```python
from build123d import *

# Parameters (mm, degrees)
SKETCH1_W                             = 12.7
SKETCH1_H                             = 50.8
BOSS_EXTRUDE1_DEPTH                   = 228.6
F_1_4_20_TAPPED_HOLE1_D               = 5.1054
F_1_4_20_TAPPED_HOLE1_DEPTH           = 19.05
F_1_4_20_TAPPED_HOLE1_TIP             = 1.533816902
F_1_4_20_TAPPED_HOLE1_ON_FACE_2_D     = 5.1054
F_1_4_20_TAPPED_HOLE1_ON_FACE_2_DEPTH = 19.05
F_1_4_20_TAPPED_HOLE1_ON_FACE_2_TIP   = 1.533816902
CUT_EXTRUDE1_DEPTH                    = 9.525
CUT_EXTRUDE2_DEPTH                    = 235.370061281
CUT_EXTRUDE3_DEPTH                    = 235.52055347


with BuildPart() as part:
    # Sketch1 → Boss-Extrude1 (new, symmetric)
    with BuildSketch(Plane(origin=(0, 0, 0), x_dir=(0, 0, -1), z_dir=(1, 0, 0))):
        with Locations((6.35, 25.4)):
            Rectangle(SKETCH1_W, SKETCH1_H)
    extrude(amount=BOSS_EXTRUDE1_DEPTH, both=True)

    # 1/4-20 Tapped Hole1
    with Locations(Plane(origin=(228.6, 41.275, -6.35), x_dir=(0, 0, 1), z_dir=(1, 0, 0))):
        with Locations((0, 0), (0, 31.75)):
            Hole(F_1_4_20_TAPPED_HOLE1_D / 2, depth=F_1_4_20_TAPPED_HOLE1_DEPTH)
            with Locations((0, 0, -(F_1_4_20_TAPPED_HOLE1_DEPTH + F_1_4_20_TAPPED_HOLE1_TIP / 2))):  # 118° drill point
                Cone(0, F_1_4_20_TAPPED_HOLE1_D / 2, F_1_4_20_TAPPED_HOLE1_TIP, mode=Mode.SUBTRACT)

    # 1/4-20 Tapped Hole1 on face 2
    with Locations(Plane(origin=(-228.6, 9.525, -6.35), x_dir=(0, 0, -1), z_dir=(-1, 0, 0))):
        with Locations((0, 0), (0, -31.75)):
            Hole(F_1_4_20_TAPPED_HOLE1_ON_FACE_2_D / 2, depth=F_1_4_20_TAPPED_HOLE1_ON_FACE_2_DEPTH)
            with Locations((0, 0, -(F_1_4_20_TAPPED_HOLE1_ON_FACE_2_DEPTH + F_1_4_20_TAPPED_HOLE1_ON_FACE_2_TIP / 2))):  # 118° drill point
                Cone(0, F_1_4_20_TAPPED_HOLE1_ON_FACE_2_D / 2, F_1_4_20_TAPPED_HOLE1_ON_FACE_2_TIP, mode=Mode.SUBTRACT)

    # Sketch4 → Cut-Extrude1 (cut)
    with BuildSketch(Plane(origin=(0, 0, -12.7), x_dir=(-1, 0, 0), z_dir=(0, 0, -1))):
        with BuildLine():
            Line((200.025, 47.625), (-200.025, 47.625))
            ThreePointArc((-200.025, 47.625), (-202.27006403, 46.69506403), (-203.2, 44.45))
            Line((-203.2, 44.45), (-203.2, 6.35))
            ThreePointArc((-203.2, 6.35), (-202.27006403, 4.10493597), (-200.025, 3.175))
            Line((-200.025, 3.175), (200.025, 3.175))
            ThreePointArc((200.025, 3.175), (202.27006403, 4.10493597), (203.2, 6.35))
            Line((203.2, 6.35), (203.2, 44.45))
            ThreePointArc((203.2, 44.45), (202.27006403, 46.69506403), (200.025, 47.625))
        make_face()
    extrude(amount=-CUT_EXTRUDE1_DEPTH, mode=Mode.SUBTRACT)

    # Sketch5 → Cut-Extrude2 (cut, through all)
    with BuildSketch(Plane(origin=(0, 0, -3.175), x_dir=(-1, 0, 0), z_dir=(0, 0, -1))):
        with BuildLine():
            Line((-200.025, 41.275), (-200.025, 9.525))
            ThreePointArc((-200.025, 9.525), (-199.09506403, 7.27993597), (-196.85, 6.35))
            Line((-196.85, 6.35), (-172.079670497, 6.35))
            ThreePointArc((-172.079670497, 6.35), (-169.226482862, 8.132180803), (-169.576379466, 11.477987203))
            Line((-169.576379466, 11.477987203), (-194.346708969, 43.227987203))
            ThreePointArc((-194.346708969, 43.227987203), (-197.882636426, 44.277380224), (-200.025, 41.275))
        make_face()
        with BuildLine():
            Line((-183.245495534, 39.322012797), (-158.475166031, 7.572012797))
            ThreePointArc((-158.475166031, 7.572012797), (-154.939238574, 6.522619776), (-152.796875, 9.525))
            Line((-152.796875, 9.525), (-152.796875, 41.275))
            ThreePointArc((-152.796875, 41.275), (-153.72681097, 43.52006403), (-155.971875, 44.45))
            Line((-155.971875, 44.45), (-180.742204503, 44.45))
            ThreePointArc((-180.742204503, 44.45), (-183.595392138, 42.667819197), (-183.245495534, 39.322012797))
        make_face()
        with BuildLine():
            Line((-149.621875, 41.275), (-149.621875, 9.525))
            ThreePointArc((-149.621875, 9.525), (-148.69193903, 7.27993597), (-146.446875, 6.35))
            Line((-146.446875, 6.35), (-121.676545497, 6.35))
            ThreePointArc((-121.676545497, 6.35), (-118.823357862, 8.132180803), (-119.173254466, 11.477987203))
            Line((-119.173254466, 11.477987203), (-143.943583969, 43.227987203))
            ThreePointArc((-143.943583969, 43.227987203), (-147.479511426, 44.277380224), (-149.621875, 41.275))
        make_face()
        with BuildLine():
            Line((-132.842370534, 39.322012797), (-108.072041031, 7.572012797))
            ThreePointArc((-108.072041031, 7.572012797), (-104.536113574, 6.522619776), (-102.39375, 9.525))
            Line((-102.39375, 9.525), (-102.39375, 41.275))
            ThreePointArc((-102.39375, 41.275), (-103.32368597, 43.52006403), (-105.56875, 44.45))
            Line((-105.56875, 44.45), (-130.339079503, 44.45))
            ThreePointArc((-130.339079503, 44.45), (-133.192267138, 42.667819197), (-132.842370534, 39.322012797))
        make_face()
        with BuildLine():
            Line((-99.21875, 41.275), (-99.21875, 9.525))
            ThreePointArc((-99.21875, 9.525), (-98.28881403, 7.27993597), (-96.04375, 6.35))
            Line((-96.04375, 6.35), (-71.273420497, 6.35))
            ThreePointArc((-71.273420497, 6.35), (-68.420232862, 8.132180803), (-68.770129466, 11.477987203))
            Line((-68.770129466, 11.477987203), (-93.540458969, 43.227987203))
            ThreePointArc((-93.540458969, 43.227987203), (-97.076386426, 44.277380224), (-99.21875, 41.275))
        make_face()
        with BuildLine():
            Line((-82.439245534, 39.322012797), (-57.668916031, 7.572012797))
            ThreePointArc((-57.668916031, 7.572012797), (-54.132988574, 6.522619776), (-51.990625, 9.525))
            Line((-51.990625, 9.525), (-51.990625, 41.275))
            ThreePointArc((-51.990625, 41.275), (-52.92056097, 43.52006403), (-55.165625, 44.45))
            Line((-55.165625, 44.45), (-79.935954503, 44.45))
            ThreePointArc((-79.935954503, 44.45), (-82.789142138, 42.667819197), (-82.439245534, 39.322012797))
        make_face()
        with BuildLine():
            Line((-48.815625, 41.275), (-48.815625, 9.525))
            ThreePointArc((-48.815625, 9.525), (-47.88568903, 7.27993597), (-45.640625, 6.35))
            Line((-45.640625, 6.35), (-20.870295497, 6.35))
            ThreePointArc((-20.870295497, 6.35), (-18.017107862, 8.132180803), (-18.367004466, 11.477987203))
            Line((-18.367004466, 11.477987203), (-43.137333969, 43.227987203))
            ThreePointArc((-43.137333969, 43.227987203), (-46.673261426, 44.277380224), (-48.815625, 41.275))
        make_face()
        with BuildLine():
            Line((-32.036120534, 39.322012797), (-7.265791031, 7.572012797))
            ThreePointArc((-7.265791031, 7.572012797), (-3.729863574, 6.522619776), (-1.5875, 9.525))
            Line((-1.5875, 9.525), (-1.5875, 41.275))
            ThreePointArc((-1.5875, 41.275), (-2.51743597, 43.52006403), (-4.7625, 44.45))
            Line((-4.7625, 44.45), (-29.532829503, 44.45))
            ThreePointArc((-29.532829503, 44.45), (-32.386017138, 42.667819197), (-32.036120534, 39.322012797))
        make_face()
        with BuildLine():
            Line((1.5875, 41.275), (1.5875, 9.525))
            ThreePointArc((1.5875, 9.525), (2.51743597, 7.27993597), (4.7625, 6.35))
            Line((4.7625, 6.35), (29.532829503, 6.35))
            ThreePointArc((29.532829503, 6.35), (32.386017138, 8.132180803), (32.036120534, 11.477987203))
            Line((32.036120534, 11.477987203), (7.265791031, 43.227987203))
            ThreePointArc((7.265791031, 43.227987203), (3.729863574, 44.277380224), (1.5875, 41.275))
        make_face()
        with BuildLine():
            Line((18.367004466, 39.322012797), (43.137333969, 7.572012797))
            ThreePointArc((43.137333969, 7.572012797), (46.673261426, 6.522619776), (48.815625, 9.525))
            Line((48.815625, 9.525), (48.815625, 41.275))
            ThreePointArc((48.815625, 41.275), (47.88568903, 43.52006403), (45.640625, 44.45))
            Line((45.640625, 44.45), (20.870295497, 44.45))
            ThreePointArc((20.870295497, 44.45), (18.017107862, 42.667819197), (18.367004466, 39.322012797))
        make_face()
        with BuildLine():
            Line((51.990625, 41.275), (51.990625, 9.525))
            ThreePointArc((51.990625, 9.525), (52.92056097, 7.27993597), (55.165625, 6.35))
            Line((55.165625, 6.35), (79.935954503, 6.35))
            ThreePointArc((79.935954503, 6.35), (82.789142138, 8.132180803), (82.439245534, 11.477987203))
            Line((82.439245534, 11.477987203), (57.668916031, 43.227987203))
            ThreePointArc((57.668916031, 43.227987203), (54.132988574, 44.277380224), (51.990625, 41.275))
        make_face()
        with BuildLine():
            Line((68.770129466, 39.322012797), (93.540458969, 7.572012797))
            ThreePointArc((93.540458969, 7.572012797), (97.076386426, 6.522619776), (99.21875, 9.525))
            Line((99.21875, 9.525), (99.21875, 41.275))
            ThreePointArc((99.21875, 41.275), (98.28881403, 43.52006403), (96.04375, 44.45))
            Line((96.04375, 44.45), (71.273420497, 44.45))
            ThreePointArc((71.273420497, 44.45), (68.420232862, 42.667819197), (68.770129466, 39.322012797))
        make_face()
        with BuildLine():
            Line((102.39375, 41.275), (102.39375, 9.525))
            ThreePointArc((102.39375, 9.525), (103.32368597, 7.27993597), (105.56875, 6.35))
            Line((105.56875, 6.35), (130.339079503, 6.35))
            ThreePointArc((130.339079503, 6.35), (133.192267138, 8.132180803), (132.842370534, 11.477987203))
            Line((132.842370534, 11.477987203), (108.072041031, 43.227987203))
            ThreePointArc((108.072041031, 43.227987203), (104.536113574, 44.277380224), (102.39375, 41.275))
        make_face()
        with BuildLine():
            Line((119.173254466, 39.322012797), (143.943583969, 7.572012797))
            ThreePointArc((143.943583969, 7.572012797), (147.479511426, 6.522619776), (149.621875, 9.525))
            Line((149.621875, 9.525), (149.621875, 41.275))
            ThreePointArc((149.621875, 41.275), (148.69193903, 43.52006403), (146.446875, 44.45))
            Line((146.446875, 44.45), (121.676545497, 44.45))
            ThreePointArc((121.676545497, 44.45), (118.823357862, 42.667819197), (119.173254466, 39.322012797))
        make_face()
        with BuildLine():
            Line((152.796875, 41.275), (152.796875, 9.525))
            ThreePointArc((152.796875, 9.525), (153.72681097, 7.27993597), (155.971875, 6.35))
            Line((155.971875, 6.35), (180.742204503, 6.35))
            ThreePointArc((180.742204503, 6.35), (183.595392138, 8.132180803), (183.245495534, 11.477987203))
            Line((183.245495534, 11.477987203), (158.475166031, 43.227987203))
            ThreePointArc((158.475166031, 43.227987203), (154.939238574, 44.277380224), (152.796875, 41.275))
        make_face()
        with BuildLine():
            Line((169.576379466, 39.322012797), (194.346708969, 7.572012797))
            ThreePointArc((194.346708969, 7.572012797), (197.882636426, 6.522619776), (200.025, 9.525))
            Line((200.025, 9.525), (200.025, 41.275))
            ThreePointArc((200.025, 41.275), (199.09506403, 43.52006403), (196.85, 44.45))
            Line((196.85, 44.45), (172.079670497, 44.45))
            ThreePointArc((172.079670497, 44.45), (169.226482862, 42.667819197), (169.576379466, 39.322012797))
        make_face()
    extrude(amount=-CUT_EXTRUDE2_DEPTH, mode=Mode.SUBTRACT)

    # Sketch6 → Cut-Extrude3 (cut, through all)
    with BuildSketch(Plane.XY):
        with BuildLine():
            Line((-215.9, 31.75), (-228.6, 31.75))
            Line((-228.6, 31.75), (-228.6, 19.05))
            Line((-228.6, 19.05), (-215.9, 19.05))
            ThreePointArc((-215.9, 19.05), (-209.55, 25.4), (-215.9, 31.75))
        make_face()
        with BuildLine():
            Line((228.6, 19.05), (215.9, 19.05))
            ThreePointArc((215.9, 19.05), (209.55, 25.4), (215.9, 31.75))
            Line((215.9, 31.75), (228.6, 31.75))
            Line((228.6, 31.75), (228.6, 19.05))
        make_face()
    extrude(amount=-CUT_EXTRUDE3_DEPTH, mode=Mode.SUBTRACT)


solid = part.part
```
Input: part model. Units: mm. Frame: model coordinates. A direction names the side the tool comes from. Round coordinates to 2 decimals unless told otherwise and drop trailing zeros. Loops run counter-clockwise (first coordinate to the right, second up) from the corner with the lowest first, then second, coordinate; pieces in that order, holes last. Notation, with made-up numbers: (87, 33.25) -> (102, 33.25) arc R19 ccw to (102, 50.25) -> close; hole circle Ø8 at (29.25, 36). An arc over 180 degrees is marked (long way). Use one line per item in the form item = value. Start each with the question number.
Item 1: Contact query for flat-ended pins moving along their axis: pin 1 Ø2.5 at (y, z) = (29.5, -1) entering from -X; pin 2 Ø2.5 at (y, z) = (23, -1.5) entering from -X; pin 3 Ø2.5 at (y, z) = (24, -1.5) entering from +X. Output: stop coordinate, or through.
Item 2: Section query B-B on x = -12. Return the cut outline in (y, z) (3 decimals).
Item 3: Section query A-A on x = -63. Return the cut outline in (y, z) (3 decimals).
Item 4: Mould query, pull axis X, two halves, no side actions, for faces 1 (the face through (-181.79, 23.67, -1.61)), 2 (the face through (-228.6, 44, -8)), 3 (the face through (-16, 38, 0)). Classes: pulls with the +X half, pulls with the -X half, needs draft (parallel to the pull), parting line crosses it, or undercut.
Item 5: Set-up query: faces 4 (the face through (16, 16, -3.175)), 5 (the face through (131.385, 27.131, -1.61)), 6 (the face through (222, 31.75, -6)), 7 (the face through (-222, 31.75, -6)). Return all of +Z, -Z, +X, -X, +Y, -Y with unobstructed straight access to the full face (end or side cutting, diameter ignored); none if empty.
Item 6: Material intervals for L1, parallel to Y at x = 223.75, z = -6.35; L2, parallel to X at y = 40, z = -9.5; L3, parallel to Y at x = -4.5, z = -11.5 (3 decimals), sorted ascending. Write a range as from..to.
Ans:
q1.pin_1 = -212.48
q1.pin_2 = -210.7
q1.pin_3 = 210.13
q2.outline = (0, -12.7) -> (3.175, -12.7) -> (3.175, -3.175) -> (6.35, -3.175) -> (6.35, 0) -> (0, 0) -> close; (37.16, -3.175) -> (47.625, -3.175) -> (47.625, -12.7) -> (50.8, -12.7) -> (50.8, 0) -> (37.16, 0) -> close
q3.outline = (0, -12.7) -> (3.175, -12.7) -> (3.175, -3.175) -> (6.35, -3.175) -> (6.35, 0) -> (0, 0) -> close; (36.395, -3.175) -> (47.625, -3.175) -> (47.625, -12.7) -> (50.8, -12.7) -> (50.8, 0) -> (36.395, 0) -> close
q4.face_1 = undercut
q4.face_2 = pulls with the -X half
q4.face_3 = needs draft
q5.face_4 = -Z
q5.face_5 = +Z, -Z
q5.face_6 = +Z, -Z, +X
q5.face_7 = +Z, -Z, -X
q6.L1 = 0..6.97, 12.08..19.05, 31.75..38.72, 43.83..50.8
q6.L2 = -228.6..-203.2, 203.2..228.6
q6.L3 = 0..3.175, 47.625..50.8
